from build123d import *

# Parameters (mm, degrees)
SKETCH1_W                      = 66
SKETCH1_H                      = 31
BOSS_EXTRUDE1_DEPTH            = 31.5
SHELL1_T                       = -1.5
CUT_EXTRUDE1_REACH             = 57.157
CUT_EXTRUDE2_REACH             = 75.435
CUT_EXTRUDE2_DIRECTION_2_REACH = 75.435
SKETCH6_W                      = 3
SKETCH6_H                      = 1.5
BOSS_EXTRUDE4_DEPTH            = 3
SKETCH6_3_W                    = 3
SKETCH6_3_H                    = 1.5
BOSS_EXTRUDE5_DEPTH            = 1
MIRROR3_COPY_1_SKETCH_W        = 3
MIRROR3_COPY_1_SKETCH_H        = 1.5
MIRROR3_COPY_1_DEPTH           = 3
MIRROR3_COPY_2_SKETCH_W        = 3
MIRROR3_COPY_2_SKETCH_H        = 1.5
MIRROR3_COPY_2_DEPTH           = 1
SKETCH7_W                      = 13
SKETCH7_H                      = 14.5
SKETCH7_W_2                    = 9
SKETCH7_H_2                    = 12
BOSS_EXTRUDE8_DEPTH            = 1.5
SKETCH7_4_W                    = 9
SKETCH7_4_H                    = 12
CUT_EXTRUDE5_DEPTH             = 1.5
CUT_EXTRUDE9_REACH             = 49.215
BOSS_EXTRUDE9_DEPTH            = 2
SKETCH12_W                     = 2.25
SKETCH12_H                     = 3.25
CUT_EXTRUDE10_DEPTH            = 1.5


with BuildPart() as part:
    # Sketch1 → Boss-Extrude1 (new body)
    with BuildSketch(Plane(origin=(0, 0, 0), x_dir=(1, 0, 0), z_dir=(0, 1, 0))):
        Rectangle(SKETCH1_W, SKETCH1_H)
    extrude(amount=BOSS_EXTRUDE1_DEPTH)

    # Shell1
    shell1_openings = [part.faces().sort_by_distance(p)[0] for p in [
        (0, 15.75, 15.5),
    ]]
    offset(amount=SHELL1_T, openings=shell1_openings, kind=Kind.INTERSECTION)

    # Sketch3 → Cut-Extrude1 (cut, up to next)
    with BuildSketch(Plane(origin=(0, 0, -15.5), x_dir=(-1, 0, 0), z_dir=(0, 0, -1)), mode=Mode.PRIVATE) as cut_extrude1_sk1:
        Polygon((29.680353068, 1.5), (3.706668857, 13.25), (-3.706668857, 13.25), (-29.680353068, 1.5), align=None)
    cut_extrude1_tool1 = extrude(cut_extrude1_sk1.sketch, amount=-CUT_EXTRUDE1_REACH, mode=Mode.PRIVATE) & part.part
    # Sketch3 → Cut-Extrude1 (cut, up to next)
    with BuildSketch(Plane(origin=(0, 0, -15.5), x_dir=(-1, 0, 0), z_dir=(0, 0, -1)), mode=Mode.PRIVATE) as cut_extrude1_sk2:
        Polygon((3.706668857, 16.603652775), (3.706668857, 14.896347225), (31.5, 2.323173612), (31.5, 29.176826388), align=None)
    cut_extrude1_tool2 = extrude(cut_extrude1_sk2.sketch, amount=-CUT_EXTRUDE1_REACH, mode=Mode.PRIVATE) & part.part
    # Sketch3 → Cut-Extrude1 (cut, up to next)
    with BuildSketch(Plane(origin=(0, 0, -15.5), x_dir=(-1, 0, 0), z_dir=(0, 0, -1)), mode=Mode.PRIVATE) as cut_extrude1_sk3:
        Polygon((-31.5, 2.323173612), (-3.706668857, 14.896347225), (-3.706668857, 16.603652775), (-31.5, 29.176826388), align=None)
    cut_extrude1_tool3 = extrude(cut_extrude1_sk3.sketch, amount=-CUT_EXTRUDE1_REACH, mode=Mode.PRIVATE) & part.part
    # Sketch3 → Cut-Extrude1 (cut, up to next)
    with BuildSketch(Plane(origin=(0, 0, -15.5), x_dir=(-1, 0, 0), z_dir=(0, 0, -1)), mode=Mode.PRIVATE) as cut_extrude1_sk4:
        Polygon((-3.706668857, 18.25), (3.706668857, 18.25), (29.680353068, 30), (-29.680353068, 30), align=None)
    cut_extrude1_tool4 = extrude(cut_extrude1_sk4.sketch, amount=-CUT_EXTRUDE1_REACH, mode=Mode.PRIVATE) & part.part
    add(cut_extrude1_tool1.solids().sort_by_distance((0, 5.8515, -15.5))[0], mode=Mode.SUBTRACT)
    add(cut_extrude1_tool2.solids().sort_by_distance((-21.68175, 15.75, -15.5))[0], mode=Mode.SUBTRACT)
    add(cut_extrude1_tool3.solids().sort_by_distance((21.68175, 15.75, -15.5))[0], mode=Mode.SUBTRACT)
    add(cut_extrude1_tool4.solids().sort_by_distance((0, 25.6485, -15.5))[0], mode=Mode.SUBTRACT)

    # Sketch4 → Cut-Extrude2 (cut, up to next)
    with BuildSketch(Plane(origin=(-31.5, 0, 0), x_dir=(0, 0, -1), z_dir=(1, 0, 0)), mode=Mode.PRIVATE) as cut_extrude2_sk1:
        Polygon((-2.5, 17.224470603), (-14, 28.929827745), (-14, 2.570172255), (-2.5, 14.275529397), align=None)
    cut_extrude2_tool1 = extrude(cut_extrude2_sk1.sketch, amount=-CUT_EXTRUDE2_REACH, mode=Mode.PRIVATE) & part.part
    # Sketch4 → Cut-Extrude2 (cut, up to next)
    with BuildSketch(Plane(origin=(-31.5, 0, 0), x_dir=(0, 0, -1), z_dir=(1, 0, 0)), mode=Mode.PRIVATE) as cut_extrude2_sk2:
        Polygon((12.948602697, 30), (-12.948602697, 30), (-2.5, 19.364815112), (2.5, 19.364815112), align=None)
    cut_extrude2_tool2 = extrude(cut_extrude2_sk2.sketch, amount=-CUT_EXTRUDE2_REACH, mode=Mode.PRIVATE) & part.part
    # Sketch4 → Cut-Extrude2 (cut, up to next)
    with BuildSketch(Plane(origin=(-31.5, 0, 0), x_dir=(0, 0, -1), z_dir=(1, 0, 0)), mode=Mode.PRIVATE) as cut_extrude2_sk3:
        Polygon((-2.5, 12.135184888), (-12.948602697, 1.5), (12.948602697, 1.5), (2.5, 12.135184888), align=None)
    cut_extrude2_tool3 = extrude(cut_extrude2_sk3.sketch, amount=-CUT_EXTRUDE2_REACH, mode=Mode.PRIVATE) & part.part
    # Sketch4 → Cut-Extrude2 (cut, up to next)
    with BuildSketch(Plane(origin=(-31.5, 0, 0), x_dir=(0, 0, -1), z_dir=(1, 0, 0)), mode=Mode.PRIVATE) as cut_extrude2_sk4:
        Polygon((14, 28.929827745), (2.5, 17.224470603), (2.5, 14.275529397), (14, 2.570172255), align=None)
    cut_extrude2_tool4 = extrude(cut_extrude2_sk4.sketch, amount=-CUT_EXTRUDE2_REACH, mode=Mode.PRIVATE) & part.part
    add(cut_extrude2_tool1.solids().sort_by_distance((-31.5, 15.75, 9.780968))[0], mode=Mode.SUBTRACT)
    add(cut_extrude2_tool2.solids().sort_by_distance((-31.5, 25.881252, 0))[0], mode=Mode.SUBTRACT)
    add(cut_extrude2_tool3.solids().sort_by_distance((-31.5, 5.618748, 0))[0], mode=Mode.SUBTRACT)
    add(cut_extrude2_tool4.solids().sort_by_distance((-31.5, 15.75, -9.780968))[0], mode=Mode.SUBTRACT)

    # Sketch4 → Cut-Extrude2 direction 2 (cut, up to next)
    with BuildSketch(Plane(origin=(-31.5, 0, 0), x_dir=(0, 0, -1), z_dir=(1, 0, 0)), mode=Mode.PRIVATE) as cut_extrude2_direction_2_sk1:
        Polygon((-2.5, 17.224470603), (-14, 28.929827745), (-14, 2.570172255), (-2.5, 14.275529397), align=None)
    cut_extrude2_direction_2_tool1 = extrude(cut_extrude2_direction_2_sk1.sketch, amount=CUT_EXTRUDE2_DIRECTION_2_REACH, mode=Mode.PRIVATE) & part.part
    # Sketch4 → Cut-Extrude2 direction 2 (cut, up to next)
    with BuildSketch(Plane(origin=(-31.5, 0, 0), x_dir=(0, 0, -1), z_dir=(1, 0, 0)), mode=Mode.PRIVATE) as cut_extrude2_direction_2_sk2:
        Polygon((12.948602697, 30), (-12.948602697, 30), (-2.5, 19.364815112), (2.5, 19.364815112), align=None)
    cut_extrude2_direction_2_tool2 = extrude(cut_extrude2_direction_2_sk2.sketch, amount=CUT_EXTRUDE2_DIRECTION_2_REACH, mode=Mode.PRIVATE) & part.part
    # Sketch4 → Cut-Extrude2 direction 2 (cut, up to next)
    with BuildSketch(Plane(origin=(-31.5, 0, 0), x_dir=(0, 0, -1), z_dir=(1, 0, 0)), mode=Mode.PRIVATE) as cut_extrude2_direction_2_sk3:
        Polygon((-2.5, 12.135184888), (-12.948602697, 1.5), (12.948602697, 1.5), (2.5, 12.135184888), align=None)
    cut_extrude2_direction_2_tool3 = extrude(cut_extrude2_direction_2_sk3.sketch, amount=CUT_EXTRUDE2_DIRECTION_2_REACH, mode=Mode.PRIVATE) & part.part
    # Sketch4 → Cut-Extrude2 direction 2 (cut, up to next)
    with BuildSketch(Plane(origin=(-31.5, 0, 0), x_dir=(0, 0, -1), z_dir=(1, 0, 0)), mode=Mode.PRIVATE) as cut_extrude2_direction_2_sk4:
        Polygon((14, 28.929827745), (2.5, 17.224470603), (2.5, 14.275529397), (14, 2.570172255), align=None)
    cut_extrude2_direction_2_tool4 = extrude(cut_extrude2_direction_2_sk4.sketch, amount=CUT_EXTRUDE2_DIRECTION_2_REACH, mode=Mode.PRIVATE) & part.part
    add(cut_extrude2_direction_2_tool1.solids().sort_by_distance((-31.5, 15.75, 9.780968))[0], mode=Mode.SUBTRACT)
    add(cut_extrude2_direction_2_tool2.solids().sort_by_distance((-31.5, 25.881252, 0))[0], mode=Mode.SUBTRACT)
    add(cut_extrude2_direction_2_tool3.solids().sort_by_distance((-31.5, 5.618748, 0))[0], mode=Mode.SUBTRACT)
    add(cut_extrude2_direction_2_tool4.solids().sort_by_distance((-31.5, 15.75, -9.780968))[0], mode=Mode.SUBTRACT)

    # Sketch6 → Boss-Extrude4 (add)
    with BuildSketch(Plane(origin=(0, 15, 0), x_dir=(-1, 0, 0), z_dir=(0, -1, 0))):
        with Locations((-30, 14.75)):
            Rectangle(SKETCH6_W, SKETCH6_H)
    boss_extrude4 = extrude(amount=-BOSS_EXTRUDE4_DEPTH)

    # Sketch6<3> → Boss-Extrude5 (add)
    with BuildSketch(Plane(origin=(0, 15, 0), x_dir=(-1, 0, 0), z_dir=(0, -1, 0))):
        with Locations((-30, 13.25)):
            Rectangle(SKETCH6_3_W, SKETCH6_3_H)
    boss_extrude5 = extrude(amount=-BOSS_EXTRUDE5_DEPTH)

    # Mirror2: Boss-Extrude4, Boss-Extrude5 across plane
    add(boss_extrude4.mirror(Plane.XY))
    add(boss_extrude5.mirror(Plane.XY))

    # Mirror3: Boss-Extrude4, Boss-Extrude5 across plane
    add(boss_extrude4.mirror(Plane.ZY))
    add(boss_extrude5.mirror(Plane.ZY))

    # Mirror3 copy 1 sketch → Mirror3 copy 1 (add)
    with BuildSketch(Plane.XZ.offset(-15)):
        with Locations((-30, 14.75)):
            Rectangle(MIRROR3_COPY_1_SKETCH_W, MIRROR3_COPY_1_SKETCH_H)
    extrude(amount=-MIRROR3_COPY_1_DEPTH)

    # Mirror3 copy 2 sketch → Mirror3 copy 2 (add)
    with BuildSketch(Plane.XZ.offset(-15)):
        with Locations((-30, 13.25)):
            Rectangle(MIRROR3_COPY_2_SKETCH_W, MIRROR3_COPY_2_SKETCH_H)
    extrude(amount=-MIRROR3_COPY_2_DEPTH)

    # Sketch7 → Boss-Extrude8 (add)
    with BuildSketch(Plane(origin=(31.5, 0, 0), x_dir=(0, 0, -1), z_dir=(1, 0, 0))):
        with Locations((7.5, 22.75)):
            Rectangle(SKETCH7_W, SKETCH7_H)
        with Locations((7, 23)):
            Rectangle(SKETCH7_W_2, SKETCH7_H_2, mode=Mode.SUBTRACT)
    extrude(amount=BOSS_EXTRUDE8_DEPTH)

    # Sketch7<4> → Cut-Extrude5 (cut)
    with BuildSketch(Plane(origin=(31.5, 0, 0), x_dir=(0, 0, -1), z_dir=(1, 0, 0))):
        with Locations((7, 23)):
            Rectangle(SKETCH7_4_W, SKETCH7_4_H)
    extrude(amount=CUT_EXTRUDE5_DEPTH, mode=Mode.SUBTRACT)

    # Sketch10 → Cut-Extrude9 (cut, up to next)
    with BuildSketch(Plane.XZ.offset(-30), mode=Mode.PRIVATE) as cut_extrude9_sk1:
        Polygon((-31.5, -13.17926185), (-3.778339162, -0.8585237), (-3.778339162, 0.8585237), (-31.5, 13.17926185), (-31.5, 12.948602697), (-31.5, -12.948602697), align=None)
    cut_extrude9_tool1 = extrude(cut_extrude9_sk1.sketch, amount=-CUT_EXTRUDE9_REACH, mode=Mode.PRIVATE) & part.part
    # Sketch10 → Cut-Extrude9 (cut, up to next)
    with BuildSketch(Plane.XZ.offset(-30), mode=Mode.PRIVATE) as cut_extrude9_sk2:
        Polygon((-3.778339162, 2.5), (3.778339162, 2.5), (29.653339162, 14), (-29.653339162, 14), align=None)
    cut_extrude9_tool2 = extrude(cut_extrude9_sk2.sketch, amount=-CUT_EXTRUDE9_REACH, mode=Mode.PRIVATE) & part.part
    # Sketch10 → Cut-Extrude9 (cut, up to next)
    with BuildSketch(Plane.XZ.offset(-30), mode=Mode.PRIVATE) as cut_extrude9_sk3:
        Polygon((3.778339162, 0.8585237), (3.778339162, -0.8585237), (31.5, -13.17926185), (31.5, -1), (31.5, 12.948602697), (31.5, 13.17926185), align=None)
    cut_extrude9_tool3 = extrude(cut_extrude9_sk3.sketch, amount=-CUT_EXTRUDE9_REACH, mode=Mode.PRIVATE) & part.part
    # Sketch10 → Cut-Extrude9 (cut, up to next)
    with BuildSketch(Plane.XZ.offset(-30), mode=Mode.PRIVATE) as cut_extrude9_sk4:
        Polygon((29.653339162, -14), (3.778339162, -2.5), (-3.778339162, -2.5), (-29.653339162, -14), align=None)
    cut_extrude9_tool4 = extrude(cut_extrude9_sk4.sketch, amount=-CUT_EXTRUDE9_REACH, mode=Mode.PRIVATE) & part.part
    add(cut_extrude9_tool1.solids().sort_by_distance((-21.694312, 30, 0))[0], mode=Mode.SUBTRACT)
    add(cut_extrude9_tool2.solids().sort_by_distance((0, 30, 9.733436))[0], mode=Mode.SUBTRACT)
    add(cut_extrude9_tool3.solids().sort_by_distance((21.694312, 30, 0))[0], mode=Mode.SUBTRACT)
    add(cut_extrude9_tool4.solids().sort_by_distance((0, 30, -9.733436))[0], mode=Mode.SUBTRACT)

    # Sketch11 → Boss-Extrude9 (add)
    with BuildSketch(Plane.ZY.offset(33)):
        Polygon((13.75, 0), (7.294759025, 0), (13.75, -4.738684311), align=None)
    boss_extrude9 = extrude(amount=-BOSS_EXTRUDE9_DEPTH)

    # Mirror5: Boss-Extrude9 across plane
    add(boss_extrude9.mirror(Plane.ZY))

    # Sketch12 → Cut-Extrude10 (cut)
    with BuildSketch(Plane.XZ):
        with Locations((-19.875, 12.125)):
            Rectangle(SKETCH12_W, SKETCH12_H)
        with Locations((19.875, 12.125)):
            Rectangle(SKETCH12_W, SKETCH12_H)
    extrude(amount=-CUT_EXTRUDE10_DEPTH, mode=Mode.SUBTRACT)


solid = part.part
Geometry: final body of the model. Coordinates: model frame, mm. A direction names the side the tool comes from. Round coordinates to 2 decimals unless told otherwise and drop trailing zeros. Loops run counter-clockwise (first coordinate to the right, second up) from the corner with the lowest first, then second, coordinate; pieces in that order, holes last.
Q1. Material intervals for L1, parallel to Y at x = 7, z = -4.5; L2, parallel to X at y = 16, z = -11, sorted ascending.
Q2. Section A-A on x = -2. Return loops of the section in (y, z).
Q3. Pin query (flat end, axial travel): P1, Ø14.5, axis at x = 3.5, y = 9, coming from the +Z side; P2, Ø6, axis at x = 20, z = -3.5, coming from the +Y side; P3, Ø1.6, axis at x = -32.5, z = -1.5, coming from the -Y side. Return the tip coordinate at first contact, or that it passes through.
Q4. Section C-C on y = 27. State how many separate pieces and enclosed holes the cut face has, plus the area to 3 significant figures.
Q5. Section B-B on x = 6.5. Return loops of the section in (y, z), plus the area to 3 significant figures.
Q6. Pull-direction query (Z, two-part tool) for faces 1 (the flat face through (-32.01, -2.34, 10.48)), 2 (the flat face through (30, 17, -14)), 3 (the flat face through (0, 31, 2.5)), 4 (the flat face through (3.707, 16, -15)); classes: released by +Z, released by -Z, zero draft, split by the parting line, or undercut.
Q7. Access query for faces 5 (the flat face through (-32, 16, -14)), 6 (the flat face through (-31.5, 18, 0)), 7 (the flat face through (17.833, 30.74, 7.105)). Directions: +Z, -Z, +X, -X, +Y, -Y. A direction counts if a zero-diameter tool reaches every point of the face in a straight line with its end or side. Return the directions, or none.
Evaluation:
1. L1: y = 0 to 1.5
1. L2: x = 31.5 to 33
2. outline: (0, -15.5) - (1.5, -15.5) - (1.5, 15.5) - (0, 15.5) - close; (13.25, -15.5) - (18.25, -15.5) - (18.25, -14) - (13.25, -14) - close; (30, -15.5) - (31.5, -15.5) - (31.5, -14) - (30, -14) - close; (30, -2.5) - (31.5, -2.5) - (31.5, 2.5) - (30, 2.5) - close; (30, 14) - (31.5, 14) - (31.5, 15.5) - (30, 15.5) - close
3. P1: stops at z = -14
3. P2: stops at y = 1.5
3. P3: stops at y = 0
4. separate pieces: 10
4. enclosed holes: 0
4. area: 35.4 mm2
5. outline: (0, -15.5) - (1.5, -15.5) - (1.5, 15.5) - (0, 15.5) - close; (11.99, -15.5) - (13.63, -15.5) - (13.63, -14) - (11.99, -14) - close; (17.87, -15.5) - (19.51, -15.5) - (19.51, -14) - (17.87, -14) - close; (30, -15.5) - (31.5, -15.5) - (31.5, -14) - (30, -14) - close; (30, -3.71) - (31.5, -3.71) - (31.5, -2.07) - (30, -2.07) - close; (30, 2.07) - (31.5, 2.07) - (31.5, 3.71) - (30, 3.71) - close; (30, 14) - (31.5, 14) - (31.5, 15.5) - (30, 15.5) - close
5. area: 60.9 mm2
6. face 1: released by -Z
6. face 2: undercut
6. face 3: undercut
6. face 4: zero draft
7. face 5: -X
7. face 6: none
7. face 7: +Y
